from build123d import *

# Parameters (mm, degrees)
SKETCH1_W           = 19.05
SKETCH1_H           = 19.05
BOSS_EXTRUDE1_DEPTH = 139.7
SKETCH2_R           = 4.7625
CUT_EXTRUDE1_DEPTH  = 20.05
SKETCH3_R           = 1.5
CUT_EXTRUDE2_DEPTH  = 20.05
FILLET1_R           = 3.175


with BuildPart() as part:
    # Sketch1 → Boss-Extrude1 (new body)
    with BuildSketch(Plane(origin=(0, 0, 0), x_dir=(0, 0, -1), z_dir=(1, 0, 0))):
        Rectangle(SKETCH1_W, SKETCH1_H)
    extrude(amount=BOSS_EXTRUDE1_DEPTH)

    # Sketch2 → Cut-Extrude1 (cut, through all)
    with BuildSketch(Plane(origin=(0, 9.525, 0), x_dir=(1, 0, 0), z_dir=(0, 1, 0))):
        with Locations((114.3, 0)):
            Circle(SKETCH2_R)
    extrude(amount=-CUT_EXTRUDE1_DEPTH, mode=Mode.SUBTRACT)

    # Sketch3 → Cut-Extrude2 (cut, through all)
    with BuildSketch(Plane.XY.offset(9.525)):
        with Locations((6.35, 0)):
            Circle(SKETCH3_R)
        with Locations((57.15, 0)):
            Circle(SKETCH3_R)
    extrude(amount=-CUT_EXTRUDE2_DEPTH, mode=Mode.SUBTRACT)

    # Fillet1
    fillet1_edges = [part.edges().sort_by_distance(p)[0] for p in [
        (69.85, -9.525, 9.525),
        (69.85, 9.525, 9.525),
        (69.85, 9.525, -9.525),
        (69.85, -9.525, -9.525),
    ]]
    fillet(fillet1_edges, radius=FILLET1_R)


solid = part.part
Can you work these out from the model? Positions are in its coordinate system, mm. Give positions to 0.01 mm unless a question says otherwise; leave off trailing zeros. Loops run counter-clockwise (first coordinate to the right, second up) from the corner with the lowest first, then second, coordinate; pieces in that order, holes last. Notation, with made-up numbers: (43, 51.25) - (66, 51.25) arc R6 ccw to (66, 58.25) - close; hole circle Ø11 at (29, -12). An arc over 180 degrees is marked (long way). Answer as a JSON object with one key per item and string values.
Q1. Imagine slicing it at B-B on x = 57.15. Write out the boundary of the cut face in (y, z) (3 decimals).
Geometry says:
{"outline": "(-9.525, -6.35) arc R3.175 ccw to (-6.35, -9.525) - (-1.5, -9.525) - (-1.5, 9.525) - (-6.35, 9.525) arc R3.175 ccw to (-9.525, 6.35) - close; (1.5, -9.525) - (6.35, -9.525) arc R3.175 ccw to (9.525, -6.35) - (9.525, 6.35) arc R3.175 ccw to (6.35, 9.525) - (1.5, 9.525) - close"}
Q2. Imagine slicing it at D-D on x = 20. Write out the boundary of the cut face in (y, z) (3 decimals), plus the area to 3 significant figures.
Geometry says:
{"outline": "(-9.525, -6.35) arc R3.175 ccw to (-6.35, -9.525) - (6.35, -9.525) arc R3.175 ccw to (9.525, -6.35) - (9.525, 6.35) arc R3.175 ccw to (6.35, 9.525) - (-6.35, 9.525) arc R3.175 ccw to (-9.525, 6.35) - close", "area": "354 mm²"}
Q3. If we mould it in two halves opening along Y, with no side actions, what happens to faces 1 (the flat face through (69, -9.525, 0)), 2 (the cylindrical face through (70.83, 8.62, -8.57)), 3 (the cylindrical face through (7.736, -0.575, 0.133)), 4 (the cylindrical face through (55.96, -0.91, 0.13))? For each: pulls with the +Y half, pulls with the -Y half, needs draft (parallel to the pull), parting line crosses it, or undercut.
Geometry says:
{"face 1": "pulls with the -Y half", "face 2": "pulls with the +Y half", "face 3": "undercut", "face 4": "undercut"}
Q4. Imagine slicing it at A-A on z = 1.25. Write out the boundary of the cut face in (x, y) (3 decimals), plus the area to 3 significant figures.
Geometry says:
{"outline": "(0, -9.525) - (109.704, -9.525) - (109.704, 9.525) - (0, 9.525) - close; (118.896, -9.525) - (139.7, -9.525) - (139.7, 9.525) - (118.896, 9.525) - close; hole circle Ø3 at (6.35, 0); hole circle Ø3 at (57.15, 0)", "area": "2,470 mm²"}
Q5. Will this pin go through, and if not, where does the flat tip stop? P1, Ø5.5, axis at x = 114.3, z = 0, coming from the +Y side.
Geometry says:
{"P1": "through"}
Q6. Imagine slicing it at C-C on y = -3.75. Write out the boundary of the cut face in (x, z) (1 decimal).
Geometry says:
{"outline": "(0, -9.5) - (139.7, -9.5) - (139.7, 9.5) - (0, 9.5) - close; hole circle Ø9.5 at (114.3, 0)"}
Q7. If I drill on L1, parallel to Z at x = 114.3, y = -3.5 (1 decimal); L2, parallel to Y at x = 6.35, z = 1.5 (3 decimals); L3, parallel to X at y = -3, z = 0, over which ranges is the centre line in solid material (lowest first)?
Geometry says:
{"L1": "-9.5 to -4.8, 4.8 to 9.5", "L2": "-9.525 to -1.5, 1.5 to 9.525", "L3": "0 to 109.54, 119.06 to 139.7"}
